Can you work these out from the model? Positions are in its coordinate system, mm. Give positions to 0.01 mm unless a question says otherwise; leave off trailing zeros. Order: outer loops, then holes, each group sorted by start corner. A loop starts at its lowest first (then second) coordinate and runs counter-clockwise, first axis right, second up. Notation, with made-up numbers: (-22.5, -20) - (6.5, -20) arc R25 ccw to (6.5, 15) - close; hole circle Ø2 at (-3.75, -31.5). An arc over 180 degrees is marked (long way). Use one line per item in the form item = value. Start each with the question number.
1) We'd pull the mould along Y, two halves only. Please class faces 1 (the flat face through (188, 0, 3)), 2 (the flat face through (242.475, 42, 3)), 3 (the flat face through (310, 69, 3)): released by +Y, released by -Y, zero draft, split by the parting line, or undercut.
2) Suppose I cut it at C-C, the plane z = 4.85. State how many separate pieces and enclosed holes the cut face has, and give its area (3 significant figures).
3) For pin 1 (1.7 mm diameter, centred on y = 126, z = 3.5, fed in from -X); pin 2 (1.4 mm diameter, centred on x = 117.5, z = 1.5, fed in from -Y); pin 3 (3 mm diameter, centred on y = 107.5, z = 3.5, fed in from -X), each with a flat end and sliding along its axis, tell me the tip position at first contact or that it passes through.
4) Suppose I cut it at B-B, the plane x = 50. Write out the boundary of the cut face in (y, z).
5) Please list where these lines run through material, in increasing order: probe 1 along Y at (x, z) = (259.5, 3.05); probe 2 along Y at (x, z) = (220.5, 2.15); probe 3 along Y at (x, z) = (128, 3.95).
6) Suppose I cut it at A-A, the plane y = 70. Write out the boundary of the cut face in (x, z).
```python
from build123d import *

# Parameters (mm, degrees)
ESQUISSE1_W             = 310
ESQUISSE1_H             = 140
BOSS_EXTRU_1_DEPTH      = 6
ESQUISSE4_W             = 4.95
ESQUISSE4_H             = 5.9
ESQUISSE4_W_2           = 5.9
ESQUISSE4_H_2           = 7.9
ENL_V_MAT_EXTRU_3_DEPTH = 6
ESQUISSE5_W             = 4.95
ESQUISSE5_H             = 5.9
ENL_V_MAT_EXTRU_4_DEPTH = 6
ESQUISSE6_W             = 4.95
ESQUISSE6_H             = 5.9
ENL_V_MAT_EXTRU_5_DEPTH = 6
ENL_V_MAT_EXTRU_6_DEPTH = 6
ESQUISSE8_R             = 5
ENL_V_MAT_EXTRU_7_DEPTH = 6
ESQUISSE9_W             = 4.8
ESQUISSE9_H             = 5.6
ENL_V_MAT_EXTRU_8_DEPTH = 10


with BuildPart() as part:
    # Esquisse1 → Boss.-Extru.1 (new body)
    with BuildSketch(Plane.XY):
        with Locations((155, 70)):
            Rectangle(ESQUISSE1_W, ESQUISSE1_H)
    extrude(amount=BOSS_EXTRU_1_DEPTH)

    # Esquisse4 → Enlèv. mat.-Extru.3 (cut)
    with BuildSketch(Plane.XY.offset(6)):
        with Locations((190.025, 108.27)):
            Rectangle(ESQUISSE4_W, ESQUISSE4_H)
        with Locations((185, 79.27)):
            Rectangle(ESQUISSE4_W_2, ESQUISSE4_H_2)
        with Locations((240, 79.27)):
            Rectangle(ESQUISSE4_W_2, ESQUISSE4_H_2)
        with Locations((180.025, 108.27)):
            Rectangle(ESQUISSE4_W, ESQUISSE4_H)
        with Locations((200.025, 108.27)):
            Rectangle(ESQUISSE4_W, ESQUISSE4_H)
        with Locations((210.025, 108.27)):
            Rectangle(ESQUISSE4_W, ESQUISSE4_H)
        with Locations((220.025, 108.27)):
            Rectangle(ESQUISSE4_W, ESQUISSE4_H)
        with Locations((230.025, 108.27)):
            Rectangle(ESQUISSE4_W, ESQUISSE4_H)
        with Locations((240.025, 108.27)):
            Rectangle(ESQUISSE4_W, ESQUISSE4_H)
    extrude(amount=-ENL_V_MAT_EXTRU_3_DEPTH, mode=Mode.SUBTRACT)

    # Esquisse5 → Enlèv. mat.-Extru.4 (cut)
    with BuildSketch(Plane(origin=(0, 0, 0), x_dir=(-1, 0, 0), z_dir=(0, 0, -1))):
        with Locations((-300, 98)):
            Rectangle(ESQUISSE5_W, ESQUISSE5_H)
        with Locations((-290, 98)):
            Rectangle(ESQUISSE5_W, ESQUISSE5_H)
        with Locations((-280, 98)):
            Rectangle(ESQUISSE5_W, ESQUISSE5_H)
        with Locations((-270, 98)):
            Rectangle(ESQUISSE5_W, ESQUISSE5_H)
        with Locations((-260, 98)):
            Rectangle(ESQUISSE5_W, ESQUISSE5_H)
        with Locations((-250, 98)):
            Rectangle(ESQUISSE5_W, ESQUISSE5_H)
        with Locations((-240, 98)):
            Rectangle(ESQUISSE5_W, ESQUISSE5_H)
        with Locations((-240, 42)):
            Rectangle(ESQUISSE5_W, ESQUISSE5_H)
        with Locations((-250, 42)):
            Rectangle(ESQUISSE5_W, ESQUISSE5_H)
        with Locations((-260, 42)):
            Rectangle(ESQUISSE5_W, ESQUISSE5_H)
        with Locations((-270, 42)):
            Rectangle(ESQUISSE5_W, ESQUISSE5_H)
        with Locations((-280, 42)):
            Rectangle(ESQUISSE5_W, ESQUISSE5_H)
        with Locations((-300, 42)):
            Rectangle(ESQUISSE5_W, ESQUISSE5_H)
        with Locations((-290, 42)):
            Rectangle(ESQUISSE5_W, ESQUISSE5_H)
    extrude(amount=-ENL_V_MAT_EXTRU_4_DEPTH, mode=Mode.SUBTRACT)

    # Esquisse6 → Enlèv. mat.-Extru.5 (cut)
    with BuildSketch(Plane(origin=(0, 0, 0), x_dir=(-1, 0, 0), z_dir=(0, 0, -1))):
        with Locations((-9.975, 78.4)):
            Rectangle(ESQUISSE6_W, ESQUISSE6_H)
        with Locations((-19.975, 78.4)):
            Rectangle(ESQUISSE6_W, ESQUISSE6_H)
        with Locations((-9.975, 61.6)):
            Rectangle(ESQUISSE6_W, ESQUISSE6_H)
        with Locations((-19.975, 61.6)):
            Rectangle(ESQUISSE6_W, ESQUISSE6_H)
    extrude(amount=-ENL_V_MAT_EXTRU_5_DEPTH, mode=Mode.SUBTRACT)

    # Esquisse7 → Enlèv. mat.-Extru.6 (cut)
    with BuildSketch(Plane(origin=(0, 0, 0), x_dir=(-1, 0, 0), z_dir=(0, 0, -1))):
        with BuildLine():
            Line((-70, 140), (0, 140))
            Line((0, 140), (30, 140))
            Line((30, 140), (30, 0))
            Line((30, 0), (0, 0))
            Line((0, 0), (-70, 0))
            ThreePointArc((-70, 0), (0, 70), (-70, 140))
        make_face()
    extrude(amount=-ENL_V_MAT_EXTRU_6_DEPTH, mode=Mode.SUBTRACT)

    # Esquisse8 → Enlèv. mat.-Extru.7 (cut)
    with BuildSketch(Plane.XY.offset(6)):
        with Locations((50, 70)):
            Circle(ESQUISSE8_R)
    extrude(amount=-ENL_V_MAT_EXTRU_7_DEPTH, mode=Mode.SUBTRACT)

    # Esquisse9 → Enlèv. mat.-Extru.8 (cut)
    with BuildSketch(Plane.XY.offset(6)):
        with Locations((117.6, 127.2)):
            Rectangle(ESQUISSE9_W, ESQUISSE9_H)
        with Locations((127.6, 127.2)):
            Rectangle(ESQUISSE9_W, ESQUISSE9_H)
        with Locations((137.6, 127.2)):
            Rectangle(ESQUISSE9_W, ESQUISSE9_H)
        with Locations((147.6, 127.2)):
            Rectangle(ESQUISSE9_W, ESQUISSE9_H)
        with Locations((157.6, 127.2)):
            Rectangle(ESQUISSE9_W, ESQUISSE9_H)
        with Locations((167.6, 127.2)):
            Rectangle(ESQUISSE9_W, ESQUISSE9_H)
    extrude(amount=-ENL_V_MAT_EXTRU_8_DEPTH, mode=Mode.SUBTRACT)


solid = part.part
```
Result sheet:
q1.face_1 = released by -Y
q1.face_2 = undercut
q1.face_3 = zero draft
q2.separate_pieces = 1
q2.enclosed_holes = 34
q2.area = 40,200 mm²
q3.pin_1 = 26.89
q3.pin_2 = 0
q3.pin_3 = 9.97
q4.outline = (2.92, 0) - (65, 0) - (65, 6) - (2.92, 6) - close; (75, 0) - (137.08, 0) - (137.08, 6) - (75, 6) - close
q5.probe_1 = 0 to 39.05, 44.95 to 95.05, 100.95 to 140
q5.probe_2 = 0 to 105.32, 111.22 to 140
q5.probe_3 = 0 to 124.4, 130 to 140
q6.outline = (0, 0) - (45, 0) - (45, 6) - (0, 6) - close; (55, 0) - (310, 0) - (310, 6) - (55, 6) - close
